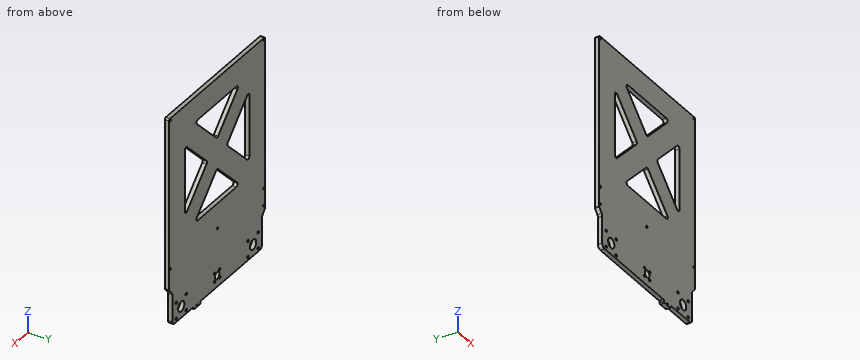
```python
from build123d import *

# Parameters (mm, degrees)
SKETCH_1_R      = 1.25
SKETCH_1_R_2    = 1.5
SKETCH_1_R_3    = 1.65
SKETCH_1_R_4    = 5
SKETCH_1_R_5    = 1.75
SKETCH_1_R_6    = 7
SKETCH_1_R_7    = 1.3
EXTRUDE_1_DEPTH = 6


with BuildPart() as part:
    # Эскиз1 → Бобышка-Вытянуть1 (new body)
    with BuildSketch(Plane(origin=(0, 0, 0), x_dir=(1, 0, 0), z_dir=(0, 1, 0))):
        with BuildLine():
            Line((96.263031015, 98.068479993), (96.263031015, 136.192066055))
            ThreePointArc((96.263031015, 136.192066055), (94.798564921, 139.727599961), (91.263031015, 141.192066055))
            Line((91.263031015, 141.192066055), (50.263031015, 141.192066055))
            ThreePointArc((50.263031015, 141.192066055), (49.202370843, 141.631405883), (48.763031015, 142.692066055))
            Line((48.763031015, 142.692066055), (48.763031015, 143.392066055))
            ThreePointArc((48.763031015, 143.392066055), (48.323691187, 144.452726227), (47.263031015, 144.892066055))
            Line((47.263031015, 144.892066055), (35.263031015, 144.892066055))
            ThreePointArc((35.263031015, 144.892066055), (34.202370843, 144.452726227), (33.763031015, 143.392066055))
            Line((33.763031015, 143.392066055), (33.763031015, 142.692066055))
            ThreePointArc((33.763031015, 142.692066055), (33.323691187, 141.631405883), (32.263031015, 141.192066055))
            Line((32.263031015, 141.192066055), (-98.736968985, 141.192066055))
            ThreePointArc((-98.736968985, 141.192066055), (-102.272502891, 139.727599961), (-103.736968985, 136.192066055))
            Line((-103.736968985, 136.192066055), (-103.736968985, 108.992066055))
            Line((-103.736968985, 108.992066055), (-103.736968985, 102.492066055))
            Line((-103.736968985, 102.492066055), (-103.736968985, 98.068479993))
            ThreePointArc((-103.736968985, 98.068479993), (-104.055758459, 96.311702257), (-104.971476189, 94.778941422))
            Line((-104.971476189, 94.778941422), (-110.214131063, 88.777741336))
            ThreePointArc((-110.214131063, 88.777741336), (-110.580418155, 88.164637002), (-110.707933945, 87.461925907))
            Line((-110.707933945, 87.461925907), (-110.707933945, -150.307933945))
            ThreePointArc((-110.707933945, -150.307933945), (-110.122147507, -151.722147507), (-108.707933945, -152.307933945))
            Line((-108.707933945, -152.307933945), (101.292066055, -152.307933945))
            ThreePointArc((101.292066055, -152.307933945), (102.706279617, -151.722147507), (103.292066055, -150.307933945))
            Line((103.292066055, -150.307933945), (103.292066055, 87.395453829))
            ThreePointArc((103.292066055, 87.395453829), (103.164550265, 88.098164923), (102.798263173, 88.711269257))
            Line((102.798263173, 88.711269257), (97.49753822, 94.778941422))
            ThreePointArc((97.49753822, 94.778941422), (96.581820489, 96.311702258), (96.263031015, 98.068479993))
        make_face()
        with Locations((-107.485559607, 83.246576588)):
            Circle(SKETCH_1_R, mode=Mode.SUBTRACT)
        with Locations((-108.207933945, -149.807933945)):
            Circle(SKETCH_1_R_2, mode=Mode.SUBTRACT)
        with Locations((100.792066055, -149.807933945)):
            Circle(SKETCH_1_R_2, mode=Mode.SUBTRACT)
        with Locations((2.042066055, 131.042066055)):
            Circle(SKETCH_1_R_3, mode=Mode.SUBTRACT)
        with Locations((-9.457933945, 131.042066055)):
            Circle(SKETCH_1_R_3, mode=Mode.SUBTRACT)
        with Locations((-4.430308283, 59.192066055)):
            Circle(SKETCH_1_R_2, mode=Mode.SUBTRACT)
        with Locations((-3.707933945, 125.292066055)):
            Circle(SKETCH_1_R_4, mode=Mode.SUBTRACT)
        with Locations((-72.394225446, 113.878357556)):
            Circle(SKETCH_1_R_5, mode=Mode.SUBTRACT)
        with Locations((-95.021642444, 136.505774554)):
            Circle(SKETCH_1_R_5, mode=Mode.SUBTRACT)
        with Locations((-83.707933945, 125.192066055)):
            Circle(SKETCH_1_R_6, mode=Mode.SUBTRACT)
        with Locations((-72.394225446, 136.505774554)):
            Circle(SKETCH_1_R_5, mode=Mode.SUBTRACT)
        with Locations((-95.021642444, 113.878357556)):
            Circle(SKETCH_1_R_5, mode=Mode.SUBTRACT)
        with Locations((87.605774554, 136.505774554)):
            Circle(SKETCH_1_R_5, mode=Mode.SUBTRACT)
        with Locations((76.292066055, 125.192066055)):
            Circle(SKETCH_1_R_6, mode=Mode.SUBTRACT)
        with Locations((64.978357556, 136.505774554)):
            Circle(SKETCH_1_R_5, mode=Mode.SUBTRACT)
        with Locations((87.605774554, 113.878357556)):
            Circle(SKETCH_1_R_5, mode=Mode.SUBTRACT)
        with Locations((-9.457933945, 119.542066055)):
            Circle(SKETCH_1_R_3, mode=Mode.SUBTRACT)
        with Locations((2.042066055, 119.542066055)):
            Circle(SKETCH_1_R_3, mode=Mode.SUBTRACT)
        with Locations((41.292066055, 142.692066055)):
            Circle(SKETCH_1_R_7, mode=Mode.SUBTRACT)
        with Locations((64.978357556, 113.878357556)):
            Circle(SKETCH_1_R_5, mode=Mode.SUBTRACT)
        with Locations((100.792066055, 59.192066055)):
            Circle(SKETCH_1_R_2, mode=Mode.SUBTRACT)
        with Locations((-108.207933945, 59.192066055)):
            Circle(SKETCH_1_R_2, mode=Mode.SUBTRACT)
        with BuildLine():
            Line((-46.524312559, 24.192066055), (39.306332642, 24.192066055))
            ThreePointArc((39.306332642, 24.192066055), (42.081691212, 22.331094066), (41.413806743, 19.056989261))
            Line((41.413806743, 19.056989261), (-1.577925667, -23.378937563))
            ThreePointArc((-1.577925667, -23.378937563), (-3.688070318, -24.243859581), (-5.796671746, -23.375182104))
            Line((-5.796671746, -23.375182104), (-48.635584538, 19.060744721))
            ThreePointArc((-48.635584538, 19.060744721), (-49.298656086, 22.333564193), (-46.524312559, 24.192066055))
        make_face(mode=Mode.SUBTRACT)
        with BuildLine():
            Line((-75.707933945, -3.543412827), (-75.707933945, -89.374058029))
            ThreePointArc((-75.707933945, -89.374058029), (-73.86499438, -92.141947324), (-70.600459844, -91.509134823))
            Line((-70.600459844, -91.509134823), (-27.200463349, -48.670222031))
            ThreePointArc((-27.200463349, -48.670222031), (-26.307938638, -46.537815787), (-27.19666547, -44.403823902))
            Line((-27.19666547, -44.403823902), (-70.596661966, -1.412091493))
            ThreePointArc((-70.596661966, -1.412091493), (-73.862529992, -0.774494633), (-75.707933945, -3.543412827))
        make_face(mode=Mode.SUBTRACT)
        with BuildLine():
            Line((-46.722200532, -117.307933945), (39.10844467, -117.307933945))
            ThreePointArc((39.10844467, -117.307933945), (41.882788196, -115.449432083), (41.219716649, -112.17661261))
            Line((41.219716649, -112.17661261), (-1.619196144, -69.740685786))
            ThreePointArc((-1.619196144, -69.740685786), (-3.727797572, -68.872008309), (-5.837942223, -69.736930327))
            Line((-5.837942223, -69.736930327), (-48.829674632, -112.172857151))
            ThreePointArc((-48.829674632, -112.172857151), (-49.497559102, -115.446961956), (-46.722200532, -117.307933945))
        make_face(mode=Mode.SUBTRACT)
        with BuildLine():
            Line((68.292066055, -3.741809861), (68.292066055, -89.572455062))
            ThreePointArc((68.292066055, -89.572455062), (66.446662102, -92.341373257), (63.180794076, -91.703776397))
            Line((63.180794076, -91.703776397), (19.78079758, -48.712043988))
            ThreePointArc((19.78079758, -48.712043988), (18.892070748, -46.578052103), (19.784595459, -44.445645859))
            Line((19.784595459, -44.445645859), (63.184591955, -1.606733067))
            ThreePointArc((63.184591955, -1.606733067), (66.44912649, -0.973920566), (68.292066055, -3.741809861))
        make_face(mode=Mode.SUBTRACT)
    extrude(amount=EXTRUDE_1_DEPTH)


solid = part.part
```
Verification items for the finished model (mm, model axes). Round coordinates to 2 decimals unless told otherwise and drop trailing zeros. Order: outer loops, then holes, each group sorted by start corner. A loop starts at its lowest first (then second) coordinate and runs counter-clockwise, first axis right, second up.
1) Material ranges on line 1 (Z direction, x = 77, y = 3.25); line 2 (X direction, y = 4.9, z = 51); line 3 (Z direction, x = 66.5, y = 3.9), recorded low to high.
Geometry says:
line 1: z = -141.19 to -132.16, -118.23 to 152.31
line 2: x = -110.71 to -75.71, -29.56 to 22.09, 68.29 to 103.29
line 3: z = -141.19 to -137.37, -135.64 to -114.74, -113.01 to 1, 92.32 to 152.31
2) Depth check by flat-ended pin: pin 1 (1.8 mm diameter, centred on y = 4, z = -114, fed in from -X). Enter the tip coordinate at first touch or a pass-through.
Geometry says:
pin 1: stops at x = -103.74
3) Cross-section at B-B, the plane x = 9. Record the cut outline in (y, z), plus the area to 3 significant figures.
Geometry says:
outline: (0, -141.19) - (6, -141.19) - (6, -24.19) - (0, -24.19) - close; (0, 12.94) - (6, 12.94) - (6, 80.26) - (0, 80.26) - close; (0, 117.31) - (6, 117.31) - (6, 152.31) - (0, 152.31) - close
area: 1,320 mm2
4) Cross-section at C-C, the plane y = 3.05. Give the number of separate pieces and of enclosed holes in the cut face, plus the area to 3 significant figures.
Geometry says:
separate pieces: 1
enclosed holes: 26
area: 51,700 mm2
5) Cross-section at A-A, the plane z = 40.5. Record the cut outline in (x, y).
Geometry says:
outline: (-110.71, 0) - (-75.71, 0) - (-75.71, 6) - (-110.71, 6) - close; (-31.14, 0) - (23.78, 0) - (23.78, 6) - (-31.14, 6) - close; (68.29, 0) - (103.29, 0) - (103.29, 6) - (68.29, 6) - close
